```python
from build123d import *

# Parameters (mm, degrees)
F0_W     = 25.4
F0_H     = 25.4
F0_W_2   = 5.953182
F0_H_2   = 3.095396
F1_DEPTH = 25.4


with BuildPart() as f1:
    # F0 (on Front) → F1 (new body)
    with BuildSketch(Plane.XZ):
        with Locations((-40.640003, -36.830003)):
            Rectangle(F0_W, F0_H)
        with Locations((-40.975282, -44.996828)):
            Rectangle(F0_W_2, F0_H_2, mode=Mode.SUBTRACT)
        Polygon((-37.998691, -40.234677), (-43.951873, -40.234677), (-43.951873, -35.948742), (-37.998691, -35.948742), (-37.998691, -31.067541), (-43.951873, -31.067541), (-47.761906, -31.067541), (-47.761906, -27.376875), (-43.951873, -27.376875), (-37.998691, -27.376875), (-32.521766, -27.376875), (-32.521766, -31.067541), (-32.521766, -35.948742), (-32.521766, -40.115625), (-37.998691, -40.115625), align=None, mode=Mode.SUBTRACT)
    extrude(amount=F1_DEPTH)


solid = f1.part
```
The listing builds one solid part. Answer for the finished solid, in the listing's coordinates (mm). A direction names the side the tool comes from. Round coordinates to 2 decimals unless told otherwise and drop trailing zeros. Loops run counter-clockwise (first coordinate to the right, second up) from the corner with the lowest first, then second, coordinate; pieces in that order, holes last.
1) For faces 4 (the face through (-41, -13, -49.53)), 5 (the face through (-32.522, -13, -34)), determine the directions among +Z, -Z, +X, -X, +Y, -Y from which every point of the face is accessible in a straight line to the end or side of a thin tool.
Outcome:
face 4: -Z, +X, -X, +Y, -Y
face 5: +Y, -Y
2) A cutting plane is placed at C-C on x = -40. Determine the outline of the cut face in (y, z).
Outcome:
outline: (-25.4, -49.53) - (0, -49.53) - (0, -46.54) - (-25.4, -46.54) - close; (-25.4, -43.45) - (0, -43.45) - (0, -40.23) - (-25.4, -40.23) - close; (-25.4, -35.95) - (0, -35.95) - (0, -31.07) - (-25.4, -31.07) - close; (-25.4, -27.38) - (0, -27.38) - (0, -24.13) - (-25.4, -24.13) - close
3) A cutting plane is placed at D-D on x = -46.25. Determine the outline of the cut face in (y, z), plus the area to 3 significant figures.
Outcome:
outline: (-25.4, -49.53) - (0, -49.53) - (0, -31.07) - (-25.4, -31.07) - close; (-25.4, -27.38) - (0, -27.38) - (0, -24.13) - (-25.4, -24.13) - close
area: 551 mm2
4) A cutting plane is placed at A-A on z = -38.25. Determine the outline of the cut face in (x, y), plus the area to 3 significant figures.
Outcome:
outline: (-53.34, -25.4) - (-43.95, -25.4) - (-43.95, 0) - (-53.34, 0) - close; (-32.52, -25.4) - (-27.94, -25.4) - (-27.94, 0) - (-32.52, 0) - close
area: 355 mm2
5) Consider line 1 (X direction, y = -19, z = -46.25); line 2 (Z direction, x = -39.5, y = -21.5); line 3 (X direction, y = -9.5, z = -27.75). Determine where each line is inside the solid, lowest interval first.
Outcome:
line 1: x = -53.34 to -43.95, -38 to -27.94
line 2: z = -49.53 to -46.54, -43.45 to -40.23, -35.95 to -31.07, -27.38 to -24.13
line 3: x = -53.34 to -47.76, -32.52 to -27.94
6) For a pull along X with two mould halves and no side action, classify faces 1 (the face through (-27.94, -13, -37)), 2 (the face through (-41, -25.4, -34)), 3 (the face through (-37.999, -13, -45)) as released by +X, released by -X, zero draft, split by the parting line, or undercut.
Outcome:
face 1: released by +X
face 2: zero draft
face 3: undercut
7) A cutting plane is placed at B-B on y = -13.5. Determine the outline of the cut face in (x, z), plus the area to 3 significant figures.
Outcome:
outline: (-53.34, -49.53) - (-27.94, -49.53) - (-27.94, -24.13) - (-53.34, -24.13) - close; hole (-47.76, -31.07) - (-38, -31.07) - (-38, -35.95) - (-43.95, -35.95) - (-43.95, -40.23) - (-38, -40.23) - (-38, -40.12) - (-32.52, -40.12) - (-32.52, -27.38) - (-47.76, -27.38) - close; hole (-43.95, -46.54) - (-38, -46.54) - (-38, -43.45) - (-43.95, -43.45) - close
area: 495 mm2
